```python
from build123d import *

# Parameters (mm, degrees)
CROQUIS1_W                 = 125
CROQUIS1_H                 = 168
SALIENTE_EXTRUIR1_DEPTH    = 5
CROQUIS2_W                 = 5
CROQUIS2_H                 = 168
SALIENTE_EXTRUIR2_DEPTH    = 75
CROQUIS3_W                 = 5
CROQUIS3_H                 = 168
SALIENTE_EXTRUIR3_DEPTH    = 75
CROQUIS4_W                 = 168
CROQUIS4_H                 = 5
SALIENTE_EXTRUIR4_DEPTH    = 30
CROQUIS5_W                 = 168
CROQUIS5_H                 = 5
SALIENTE_EXTRUIR5_DEPTH    = 30
CROQUIS6_R                 = 2.5
CORTAR_EXTRUIR1_DEPTH      = 31
CORTAR_EXTRUIR1_DEPTH_BACK = 135


with BuildPart() as part:
    # Croquis1 → Saliente-Extruir1 (new body)
    with BuildSketch(Plane(origin=(0, 0, 0), x_dir=(1, 0, 0), z_dir=(0, 1, 0))):
        with Locations((62.5, 84)):
            Rectangle(CROQUIS1_W, CROQUIS1_H)
    extrude(amount=SALIENTE_EXTRUIR1_DEPTH)

    # Croquis2 → Saliente-Extruir2 (add)
    with BuildSketch(Plane(origin=(0, 5, 0), x_dir=(1, 0, 0), z_dir=(0, 1, 0))):
        with Locations((2.5, 84)):
            Rectangle(CROQUIS2_W, CROQUIS2_H)
    extrude(amount=SALIENTE_EXTRUIR2_DEPTH)

    # Croquis3 → Saliente-Extruir3 (add)
    with BuildSketch(Plane(origin=(0, 5, 0), x_dir=(1, 0, 0), z_dir=(0, 1, 0))):
        with Locations((122.5, 84)):
            Rectangle(CROQUIS3_W, CROQUIS3_H)
    extrude(amount=SALIENTE_EXTRUIR3_DEPTH)

    # Croquis4 → Saliente-Extruir4 (add)
    with BuildSketch(Plane(origin=(5, 0, 0), x_dir=(0, 0, -1), z_dir=(1, 0, 0))):
        with Locations((84, 32.5)):
            Rectangle(CROQUIS4_W, CROQUIS4_H)
    extrude(amount=SALIENTE_EXTRUIR4_DEPTH)

    # Croquis5 → Saliente-Extruir5 (add)
    with BuildSketch(Plane.ZY.offset(-120)):
        with Locations((-84, 32.5)):
            Rectangle(CROQUIS5_W, CROQUIS5_H)
    extrude(amount=SALIENTE_EXTRUIR5_DEPTH)

    # Croquis6 → Cortar-Extruir1 (cut, two sides)
    with BuildSketch(Plane.ZY) as cortar_extruir1_sk:
        with Locations((-15, 70)):
            Circle(CROQUIS6_R)
    extrude(amount=CORTAR_EXTRUIR1_DEPTH, mode=Mode.SUBTRACT)
    extrude(cortar_extruir1_sk.sketch, amount=-CORTAR_EXTRUIR1_DEPTH_BACK, mode=Mode.SUBTRACT)


solid = part.part
```
Model file for the job. Use its own axes, mm. A direction names the side the tool comes from. Coordinates: 2 decimals unless noted, no trailing zeros. Order: outer loops, then holes, each group sorted by start corner. A loop starts at its lowest first (then second) coordinate and runs counter-clockwise, first axis right, second up. Notation, with made-up numbers: (-39, -27.5) -> (4, -27.5) arc R22 cw to (4, -17.5) -> close; hole circle Ø6 at (51, 52.25). An arc over 180 degrees is marked (long way). Return JSON: item names as keys, results as strings.
Item 1: 3-axis set-ups, long thin cutter, end or side, ignore diameter. For faces 4 (the face through (90, 33, -85)), 5 (the face through (20, 30, -83)), 6 (the face through (122.46, 67.56, -15.54)): which of +Z, -Z, +X, -X, +Y, -Y reach the whole face in a straight line?
Model answer:
{"face 4": "+Z, -Z, +Y", "face 5": "+Z, -Z", "face 6": "+X, -X"}
Item 2: Slice it at B-B (x = 23). Write the cut outline in (y, z).
Model answer:
{"outline": "(0, -168) -> (5, -168) -> (5, 0) -> (0, 0) -> close; (30, -168) -> (35, -168) -> (35, 0) -> (30, 0) -> close"}
Item 3: Slice it at D-D (y = 12). Write the cut outline in (x, z), then the cut area to 3 significant figures.
Model answer:
{"outline": "(0, -168) -> (5, -168) -> (5, 0) -> (0, 0) -> close; (120, -168) -> (125, -168) -> (125, 0) -> (120, 0) -> close", "area": "1,680 mm²"}
Item 4: Slice it at A-A (z = -15). Write the cut outline in (x, y), then the cut area to 4 significant figures.
Model answer:
{"outline": "(0, 0) -> (125, 0) -> (125, 67.5) -> (120, 67.5) -> (120, 35) -> (90, 35) -> (90, 30) -> (120, 30) -> (120, 5) -> (5, 5) -> (5, 30) -> (35, 30) -> (35, 35) -> (5, 35) -> (5, 67.5) -> (0, 67.5) -> close; (0, 72.5) -> (5, 72.5) -> (5, 80) -> (0, 80) -> close; (120, 72.5) -> (125, 72.5) -> (125, 80) -> (120, 80) -> close", "area": "1,625 mm²"}
Item 5: Pin check, flat tips, straight feed: P1, Ø1.5, axis at x = 52.5, z = -18, coming from the +Y side; P2, Ø24, axis at x = 18, z = -71.5, coming from the +Y side. Stop position of each tip, or through.
Model answer:
{"P1": "stops at y = 5", "P2": "stops at y = 35"}
Item 6: Mould opens along X. For faces 1 (the face through (2, 80, -85)), 2 (the face through (125, 39, -83)), 3 (the face through (5, 17, -83)) say: pulls with the +X half, pulls with the -X half, needs draft (parallel to the pull), parting line crosses it, or undercut.
Model answer:
{"face 1": "needs draft", "face 2": "pulls with the +X half", "face 3": "undercut"}
Item 7: Slice it at C-C (y = 70). Write the cut outline in (x, z), then the cut area to 3 significant figures.
Model answer:
{"outline": "(0, -168) -> (5, -168) -> (5, -17.5) -> (0, -17.5) -> close; (0, -12.5) -> (5, -12.5) -> (5, 0) -> (0, 0) -> close; (120, -168) -> (125, -168) -> (125, -17.5) -> (120, -17.5) -> close; (120, -12.5) -> (125, -12.5) -> (125, 0) -> (120, 0) -> close", "area": "1,630 mm²"}
Item 8: Wall check: line 1 along X through (y, z) = (9.5, -148); line 2 along Y through (x, z) = (2.1, -15); line 3 along Y through (x, z) = (9.5, -73.5). Give the ranges that are in metal, low to high. Write a range as from..to.
Model answer:
{"line 1": "x = 0..5, 120..125", "line 2": "y = 0..67.5, 72.5..80", "line 3": "y = 0..5, 30..35"}
